Geometry check sheet. Reference: the model listing, model coordinates, mm. A direction names the side the tool comes from. Coordinates: 2 decimals unless noted, no trailing zeros. Write each loop counter-clockwise with the first axis right and the second up, starting at its lowest first coordinate (ties: lowest second). Pieces come first, ordered by that corner, then holes. Notation, with made-up numbers: (0.5, 88) -> (27.5, 88) arc R17 cw to (27.5, 111) -> close; hole circle Ø9 at (-4, 43.5). An arc over 180 degrees is marked (long way). Answer in a Markdown table with one row per item. Add a question column.
1. Scan lines: L1, parallel to X at y = -6.5, z = 1.6; L2, parallel to X at y = 4, z = 2.2. Record each from-to range of solid material in increasing order. Write a range as from..to.
2. Mould release check, pull along X, two halves, no side actions. Record for faces 3 (the flat face through (-38, 0, 1)), 4 (the flat face through (-2.5, 3, 2)), 5 (the flat face through (-1, 0, 0)): pulls with the +X half, pulls with the -X half, needs draft (parallel to the pull), parting line crosses it, or undercut.
3. Set-up check for faces 1 (the flat face through (0, -7.1, 2)), 2 (the flat face through (38, 0, 1)): record each of +Z, -Z, +X, -X, +Y, -Y from which the full face is reachable in a straight line by a thin tool's end or side.
4. Cross-section at A-A on z = 1.6. Record the cut outline in (x, y).
5. Depth check by flat-ended pin: P1, Ø2.5, axis at x = 12, y = 2.9, coming from the +Z side. Enter the tip coordinate at first touch or a pass-through.
Autodesk Inventor part; units mm, degrees
ref_plane "YZ Plane" through (0, 0, 0) normal (1, 0, 0) x (0, 1, 0)
ref_plane "XZ Plane" through (0, 0, 0) normal (0, 1, 0) x (-1, 0, 0)
ref_plane "XY Plane" through (0, 0, 0) normal (0, 0, 1) x (1, 0, 0)
sketch "Skizze1" plane through (0, 0, 0) normal (0, 0, 1) x (1, 0, 0)
  line L0 (38, -12.9) -> (-38, -12.9)
  line L1 (-38, -12.9) -> (-38, 12.9)
  line L2 (-38, 12.9) -> (38, 12.9)
  line L3 (38, 12.9) -> (38, -12.9)
  line L4 (38, -12.9) -> (-38, 12.9) construction
  line L5 (-38, -12.9) -> (38, 12.9) construction
  point P0 (0, 0)
  dimension "d0" = 76
  dimension "d1" = 25.8
extrude "Extrusion1" add sketch "Skizze1" along normal blind 2.5
sketch "Skizze2" plane through (0, 0, 2.5) normal (0, 0, 1) x (1, 0, 0)
  line L0 (38, 12.9) -> (-38, 12.9)
  line L1 (-38, 12.9) -> (-38, -12.9)
  line L2 (-38, -12.9) -> (38, -12.9)
  line L3 (38, -12.9) -> (38, 12.9)
  line L4 (2.5, -7.1) -> (-2.5, -7.1)
  line L5 (-2.5, -7.1) -> (-2.5, 12.9)
  line L6 (-2.5, 12.9) -> (2.5, 12.9)
  line L7 (2.5, 12.9) -> (2.5, -7.1)
  line L8 (2.5, -7.1) -> (-2.5, 12.9) construction
  line L9 (-2.5, -7.1) -> (2.5, 12.9) construction
  point P0 (0, 0)
  point P1 (0, 2.9)
  point P2 (0, 12.9)
  dimension "d4" = 5
  dimension "d5" = 20
extrude "Extrusion2" cut sketch "Skizze2" against normal blind 1.5 contours L7 L4 L5 L0
sketch "Skizze3" plane through (-38, 12.9, 0) normal (0, 1, 0) x (1, 0, 0)
  line L0 (40.5, -2.5) -> (35.5, -2.5)
  line L1 (40.5, -2.5) -> (40.5, -1)
  line L2 (40.5, -1) -> (35.5, -1)
  line L3 (35.5, -2.5) -> (35.5, -1)
  circle A0 centre (38, -2.375) radius 0.125
  point P0 (38, 0)
  dimension "d8" = 0.25
extrude "Extrusion3" add sketch "Skizze3" against normal up to surface (20 mm away) contours A0
pattern_linear "Rechteckige Anordnung1" count 11 spacing 0.25 along (-1, 0, 0) count 11 spacing 0.25 along (1, 0, 0) of "Extrusion3"
ref_plane "Arbeitsebene1" through (0, -12.9, 0) normal (1, 0, 0) x (0, 0, -1)
sketch "Skizze4" plane through (0, 0, 2.5) normal (0, 0, 1) x (1, 0, 0)
  line L0 (2.5, 12.9) -> (2.5, -7.1)
  line L1 (2.5, -7.1) -> (2.25, -7.1)
  line L2 (2.25, -7.1) -> (2, -7.1)
  line L3 (2, -7.1) -> (1.75, -7.1)
  line L4 (1.75, -7.1) -> (1.5, -7.1)
  line L5 (1.5, -7.1) -> (1.25, -7.1)
  line L6 (1.25, -7.1) -> (1, -7.1)
  line L7 (1, -7.1) -> (0.75, -7.1)
  line L8 (0.75, -7.1) -> (0.5, -7.1)
  line L9 (0.5, -7.1) -> (0.25, -7.1)
  line L10 (0.25, -7.1) -> (0, -7.1)
  line L11 (0, -7.1) -> (-0.25, -7.1)
  line L12 (-0.25, -7.1) -> (-0.5, -7.1)
  line L13 (-0.5, -7.1) -> (-0.75, -7.1)
  line L14 (-0.75, -7.1) -> (-1, -7.1)
  line L15 (-1, -7.1) -> (-1.25, -7.1)
  line L16 (-1.25, -7.1) -> (-1.5, -7.1)
  line L17 (-1.5, -7.1) -> (-1.75, -7.1)
  line L18 (-1.75, -7.1) -> (-2, -7.1)
  line L19 (-2, -7.1) -> (-2.25, -7.1)
  line L20 (-2.25, -7.1) -> (-2.5, -7.1)
  line L21 (-2.5, -7.1) -> (-2.5, 12.9)
  line L22 (-2.5, 12.9) -> (-38, 12.9)
  line L23 (-38, 12.9) -> (-38, -12.9)
  line L24 (-38, -12.9) -> (38, -12.9)
  line L25 (38, -12.9) -> (38, 12.9)
  line L26 (38, 12.9) -> (2.5, 12.9)
  circle A0 centre (-12, 2.9) radius 1.5
  line L27 (0, 18.06) -> (0, -18.06)
  circle A1 centre (12, 2.9) radius 1.5
  point P0 (0, 0)
  dimension "d17" = 3
  dimension "d18" = 12
  dimension "d19" = 10
extrude "Extrusion4" cut sketch "Skizze4" against normal blind 2.5 contours A0 | A1
properties part number "00_chipnano_waveguide_slidsize_modified"
Results found:
| question | item | result |
|---|---|---|
| 1 | L1 | x = -38..-2.5, 2.5..38 |
| 1 | L2 | x = -38..-13.02, -10.98..-2.5, 2.5..10.98, 13.02..38 |
| 2 | face 3 | pulls with the -X half |
| 2 | face 4 | undercut |
| 2 | face 5 | needs draft |
| 3 | face 1 | +Y |
| 3 | face 2 | +Z, -Z, +X, +Y, -Y |
| 4 | outline | (-38, -12.9) -> (38, -12.9) -> (38, 12.9) -> (2.5, 12.9) -> (2.5, -7.1) -> (-2.5, -7.1) -> (-2.5, 12.9) -> (-38, 12.9) -> close; hole circle Ø3 at (-12, 2.9); hole circle Ø3 at (12, 2.9) |
| 5 | P1 | passes through |
